CAD build for the part. Positions are in the model's coordinates, mm. Face numbers are marked on the shaded views. Give positions to 0.01 mm unless a question says otherwise; leave off trailing zeros. Write each loop counter-clockwise with the first axis right and the second up, starting at its lowest first coordinate (ties: lowest second). Pieces come first, ordered by that corner, then holes. Notation, with made-up numbers: (88, -22.5) -> (95, -22.5) arc R29 cw to (95, -2.5) -> close; hole circle Ø11 at (77, 61.5). An arc over 180 degrees is marked (long way). Use one line per item in the form item = value. Start each with the question number.
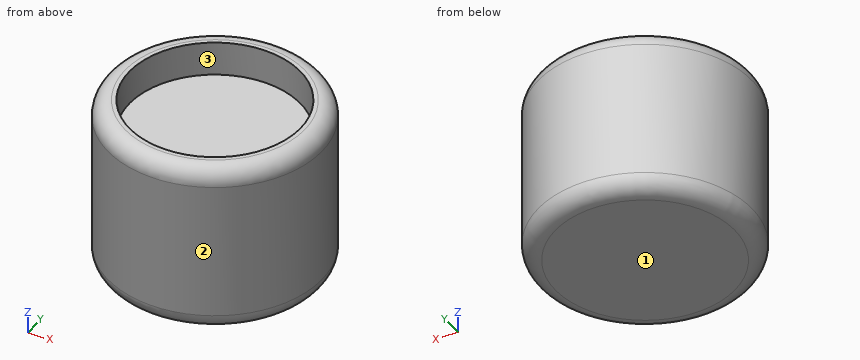
from build123d import *

# Parameters (mm, degrees)
F0_R     = 47.625
F1_DEPTH = 76.2
F4_D     = 76.2
F5_R     = 7.62
F6_R     = 7.62
F7_R     = 38.1
F8_DEPTH = 60.96


with BuildPart() as f1:
    # F0 (on Top) → F1 (new body)
    with BuildSketch(Plane.XY):
        Circle(F0_R)
    extrude(amount=F1_DEPTH)

    # F4 (through all)
    with Locations(Plane.XY.offset(76.2)):
        with Locations((0, 0)):
            Hole(F4_D / 2)

    # F5
    f5_edges = [f1.edges().sort_by_distance(p)[0] for p in [
        (-47.625, 0, 76.2),
    ]]
    fillet(f5_edges, radius=F5_R)

    # F6
    f6_edges = [f1.edges().sort_by_distance(p)[0] for p in [
        (-47.625, 0, 0),
    ]]
    fillet(f6_edges, radius=F6_R)

    # F7 (on Top) → F8 (join)
    with BuildSketch(Plane.XY):
        Circle(F7_R)
    extrude(amount=F8_DEPTH)


solid = f1.part
1) Cut at D-D (z = 5.5). Give the cut face in (x, y).
2) Two-plate mould, pull along X, no slides. Class the marked faces 1, 2 and 3: released by +X, released by -X, zero draft, split by the parting line, or undercut.
3) Pin check, flat tips, straight feed: pin 1 (6 mm diameter, centred on y = 35.5, z = 16.5, fed in from -X); pin 2 (1.5 mm diameter, centred on y = 11, z = 14.5, fed in from +X); pin 3 (2 mm diameter, centred on y = -34, z = 42, fed in from +X); pin 4 (1 mm diameter, centred on x = 21.5, y = 2.5, fed in from -Z). Stop position of each tip, or through.
4) Wall check: line 1 along Y through (x, z) = (0, 66) (3 decimals); line 2 along Z through (x, y) = (-17, 2); line 3 along Y through (x, z) = (0, 72.25). Give the ranges that are in metal, low to high. Write a range as from..to.
5) Cut at A-A (y = 0). Give the cut face in (x, z) (3 decimals), and give its area (3 significant figures).
6) Cut at C-C (z = 37). Give the cut face in (x, y) (3 decimals).
Final values:
q1.outline = circle Ø94.65 at (0, 0)
q2.face_1 = zero draft
q2.face_2 = split by the parting line
q2.face_3 = undercut
q3.pin_1 = -34.81
q3.pin_2 = 46.51
q3.pin_3 = 34.34
q3.pin_4 = 0
q4.line_1 = -47.625..-38.1, 38.1..47.625
q4.line_2 = 0..60.96
q4.line_3 = -46.68..-38.1, 38.1..46.68
q5.outline = (-47.625, 7.62) arc R7.62 ccw to (-40.005, 0) -> (40.005, 0) arc R7.62 ccw to (47.625, 7.62) -> (47.625, 68.58) arc R7.62 ccw to (40.005, 76.2) -> (38.1, 76.2) -> (38.1, 60.96) -> (-38.1, 60.96) -> (-38.1, 76.2) -> (-40.005, 76.2) arc R7.62 ccw to (-47.625, 68.58) -> close
q5.area = 6,050 mm^2
q6.outline = circle Ø95.25 at (0, 0)
